Job drawing, mm, ordinate dimensions from the low corner. One solid piece. A direction names the side the tool comes from. Coordinates: 2 decimals unless noted, no trailing zeros. Loops run counter-clockwise (first coordinate to the right, second up) from the corner with the lowest first, then second, coordinate; pieces in that order, holes last. Notation, with made-up numbers: (18.25, 56) - (33.25, 56) arc R30 ccw to (33.25, 85) - close; hole circle Ø11 at (88, 89.5). An arc over 180 degrees is marked (long way). One line per question, with ' | ' between items. Start each with the question number.
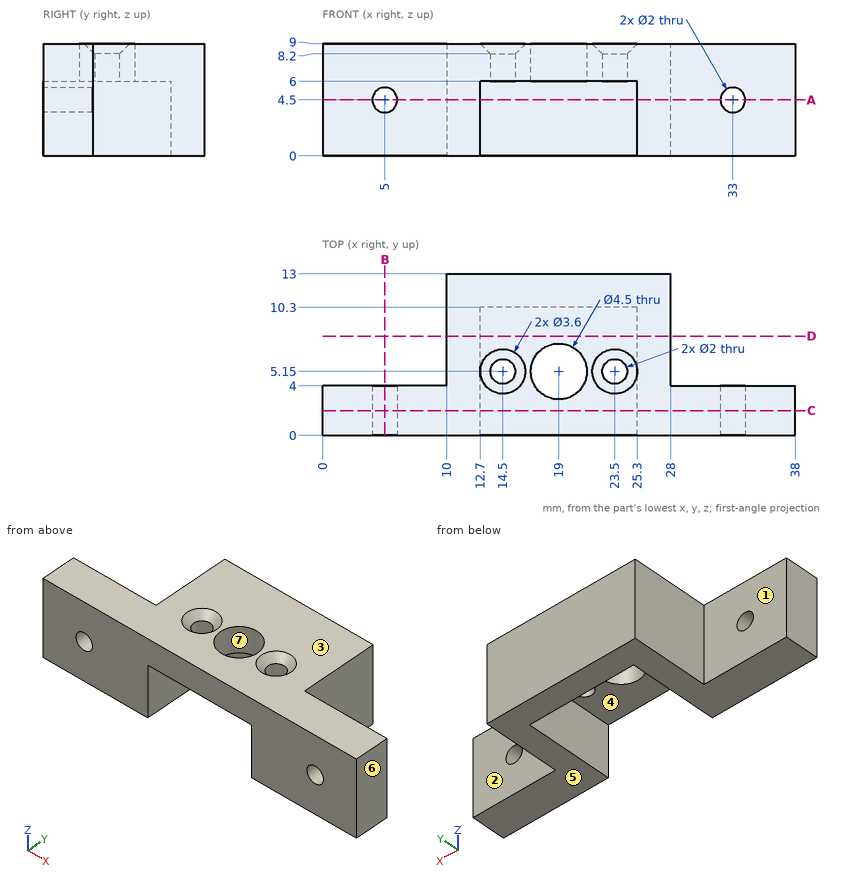
1) Band-saw the part on C-C on y = 2. List the corners of the cut face in (x, z).
2) Pin check, flat tips, straight feed: pin 1 Ø4.5 at (x, z) = (34.5, 3) entering from +Y; pin 2 Ø3 at (x, y) = (23.5, 5.15) entering from -Z; pin 3 Ø3 at (y, z) = (6, 2.5) entering from -X. Stop position of each tip, or through.
3) Wall check: line 1 along Z through (x, y) = (33, 2.75); line 2 along X through (y, z) = (8.25, 2.5); line 3 along Y through (x, z) = (19, 7.1). Give the ranges that are in metal, low to high. Write a range as [from, to].
4) Tool access for the marked faces 1, 2, 3 and 4: list every direction of +Z, -Z, +X, -X, +Y, -Y with a clear straight run to the whole face (end or side of a thin tool).
5) Band-saw the part on D-D on y = 8. List the corners of the cut face in (x, z), then the cut area to 3 significant figures.
6) Band-saw the part on A-A on z = 4.5. List the corners of the cut face in (x, y).
7) Band-saw the part on B-B on x = 5. List the corners of the cut face in (y, z).
8) Mould opens along X. For the marked faces 5, 6 and 7 say: +X half, -X half, draft (parallel to the pull), parting line (faces both ways), or undercut.
Values found:
1) outline: (0, 0) - (12.7, 0) - (12.7, 6) - (25.3, 6) - (25.3, 0) - (38, 0) - (38, 9) - (0, 9) - close; hole circle Ø2 at (5, 4.5); hole circle Ø2 at (33, 4.5)
2) pin 1: y = 4 | pin 2: z = 6 | pin 3: x = 10
3) line 1: [0, 3.5], [5.5, 9] | line 2: [10, 12.7], [25.3, 28] | line 3: [0, 2.9], [7.4, 13]
4) face 1: +Z, -Z, -X, +Y | face 2: +Z, -Z, +X, +Y | face 3: +Z, +X, -X, +Y, -Y | face 4: -Z, -Y
5) outline: (10, 0) - (12.7, 0) - (12.7, 6) - (25.3, 6) - (25.3, 0) - (28, 0) - (28, 9) - (10, 9) - close | area: 86.4 mm²
6) outline: (0, 0) - (4, 0) - (4, 4) - (0, 4) - close; (6, 0) - (12.7, 0) - (12.7, 10.3) - (25.3, 10.3) - (25.3, 0) - (32, 0) - (32, 4) - (28, 4) - (28, 13) - (10, 13) - (10, 4) - (6, 4) - close; (34, 0) - (38, 0) - (38, 4) - (34, 4) - close
7) outline: (0, 0) - (4, 0) - (4, 3.5) - (0, 3.5) - close; (0, 5.5) - (4, 5.5) - (4, 9) - (0, 9) - close
8) face 5: draft | face 6: +X half | face 7: undercut
